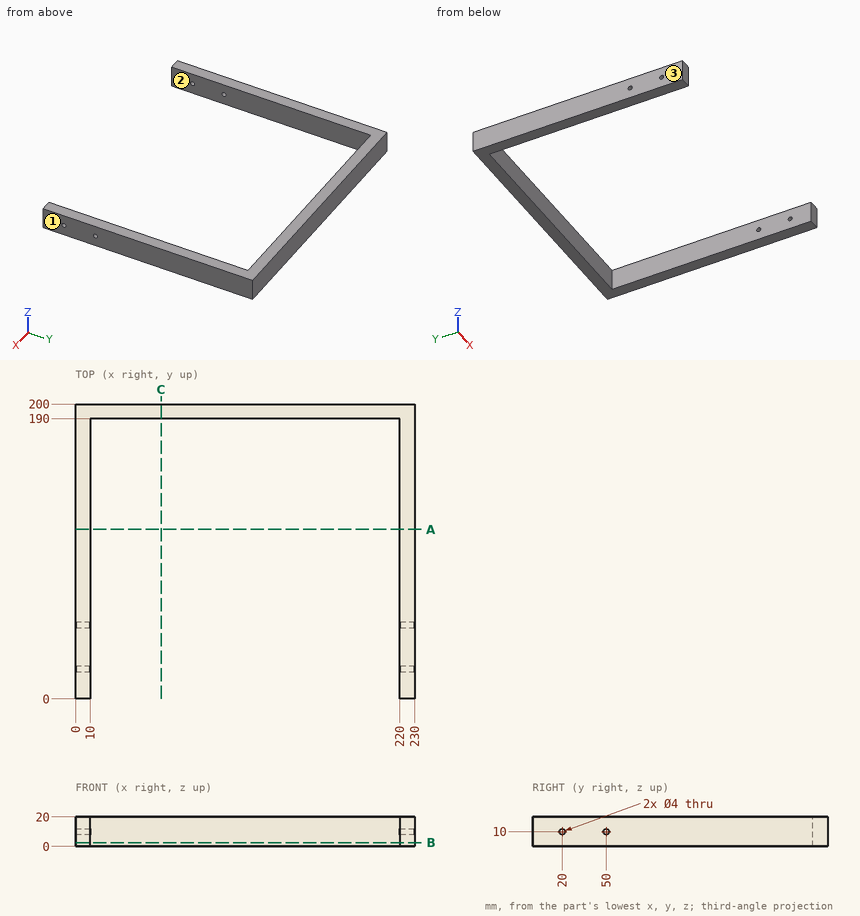
Print and shaded views of the part. All mm, measured from the part's lowest x, y and z. Give positions to 0.01 mm unless a question says otherwise; leave off trailing zeros. Write each loop counter-clockwise with the first axis right and the second up, starting at its lowest first coordinate (ties: lowest second). Pieces come first, ordered by that corner, then holes. Notation, with made-up numbers: (78.5, 24.5) -> (104.5, 24.5) arc R28 cw to (104.5, 59.5) -> close; hole circle Ø1 at (-9, 35.25). An arc over 180 degrees is marked (long way). Use CSV: the item, a comma, the result in double quotes. Start each with the question number.
1) Two-plate mould, pull along X, no slides. Class the marked faces 1, 2 and 3: released by +X, released by -X, zero draft, split by the parting line, or undercut.
2) Drill centre lines: L1, parallel to Y at x = 223.75, z = 10; L2, parallel to X at y = 154, z = 12.75; L3, parallel to Y at x = 67, z = 16.75. Where is each one in solid material? Low to high.
3) Cut at C-C on x = 58. List the corners of the cut face in (y, z).
4) Pin check, flat tips, straight feed: P1, Ø2, axis at x = 103, z = 8.5, coming from the -Y side; P2, Ø2.5, axis at y = 50, z = 10, coming from the +X side. Stop position of each tip, or through.
5) Cut at A-A on y = 115. List the corners of the cut face in (x, z).
6) Cut at B-B on z = 2.5. List the corners of the cut face in (x, y).
Final values:
1,face 1,"released by +X"
1,face 2,"undercut"
1,face 3,"released by -X"
2,L1,"y = 0 to 18, 22 to 48, 52 to 200"
2,L2,"x = 0 to 10, 220 to 230"
2,L3,"y = 190 to 200"
3,outline,"(190, 0) -> (200, 0) -> (200, 20) -> (190, 20) -> close"
4,P1,"stops at y = 190"
4,P2,"passes through"
5,outline,"(0, 0) -> (10, 0) -> (10, 20) -> (0, 20) -> close; (220, 0) -> (230, 0) -> (230, 20) -> (220, 20) -> close"
6,outline,"(0, 0) -> (10, 0) -> (10, 190) -> (220, 190) -> (220, 0) -> (230, 0) -> (230, 200) -> (0, 200) -> close"
